The listing builds one solid part. Answer for the finished solid, in the listing's coordinates (mm). Face numbers are marked on the shaded views. A direction names the side the tool comes from. Give positions to 0.01 mm unless a question says otherwise; leave off trailing zeros. Write each loop counter-clockwise with the first axis right and the second up, starting at its lowest first coordinate (ties: lowest second). Pieces come first, ordered by that corner, then holes. Notation, with made-up numbers: (-32.75, 13) - (-2.75, 13) arc R23 ccw to (-2.75, 32) - close; hole circle Ø10 at (69, 54). An arc over 180 degrees is marked (long way). Answer as CSV lines item,"result". Start each with the question number.
(1) Straight lines are drawn through the part: probe 1 along Z at (x, y) = (0, 0.1); probe 2 along Z at (x, y) = (-2, -2.25); probe 3 along Y at (x, z) = (0, 13.25). For each, find the intervals that lie inside material, in ascending order.
(2) Each of these flat-tipped pins is pushed along its axis until it touches: pin 1 Ø3 at (x, z) = (-1, 15) entering from -Y; pin 2 Ø0.7 at (y, z) = (-2, 4) entering from -X; pin 3 Ø0.7 at (y, z) = (-1, 15) entering from +X; pin 4 Ø3 at (x, z) = (0, 15.29) entering from -Y. Where does it stop, or does it pass through?
(3) Find section D-D (x = 2.5). Write down the section's boundary in (y, z), then the cut area to 3 significant figures.
(4) Find section B-B (z = 4). Write down the section's boundary in (x, y), then the cut area to 3 significant figures.
(5) For a pull along X with two mould halves and no side action, classify the marked faces 1, 2 and 3 as pulls with the +X half, pulls with the -X half, needs draft (parallel to the pull), parting line crosses it, or undercut.
(6) Find section A-A (y = -1.4). Write down the section's boundary in (x, z).
(7) Find section C-C (z = 9). Write down the section's boundary in (x, y), then the cut area to 3 significant figures.
(8) For the marked faces 4 and 5, determine the directions among +Z, -Z, +X, -X, +Y, -Y from which every point of the face is accessible in a straight line to the end or side of a thin tool.
from build123d import *

# Parameters (mm, degrees)
PAD_DEPTH       = 20
SKETCH001_W     = 5.88
SKETCH001_H     = 1.68
POCKET_DEPTH    = 20
POCKET001_DEPTH = 2.4
SKETCH003_R     = 1.6
POCKET002_DEPTH = 1.6


with BuildPart() as part:
    # Sketch → Pad (new body)
    with BuildSketch(Plane.XY):
        Polygon((2.94, -2.84), (-2.94, -2.84), (-5.44, -0.52), (-5.44, 1.16), (-2.94, 1.16), (-2.94, 2.84), (2.94, 2.84), (2.94, 1.16), (5.44, 1.16), (5.44, -0.52), align=None)
    extrude(amount=PAD_DEPTH)

    # Sketch001 (on Face11 of Pad) → Pocket (cut)
    with BuildSketch(Plane(origin=(0, 0, 0), x_dir=(1, 0, 0), z_dir=(0, 0, -1))):
        with Locations((0, -2)):
            Rectangle(SKETCH001_W, SKETCH001_H)
    extrude(amount=-POCKET_DEPTH, mode=Mode.SUBTRACT)

    # Sketch002 (on Face1 of Pocket) → Pocket001 (cut)
    with BuildSketch(Plane.XZ.offset(2.84)):
        Polygon((0, 18.6), (-2.87, 16.943005), (-2.87, 13.629014), (0, 11.972019), (2.87, 13.629014), (2.87, 16.943005), align=None)
        Polygon((2.87, 6.370986), (0, 8.027981), (-2.87, 6.370986), (-2.87, 3.056995), (0, 1.4), (2.87, 3.056995), align=None)
    extrude(amount=-POCKET001_DEPTH, mode=Mode.SUBTRACT)

    # Sketch003 (on Face24 of Pocket001) → Pocket002 (cut)
    with BuildSketch(Plane.XZ.offset(0.44)):
        with Locations((0, 15.286009)):
            Circle(SKETCH003_R)
        with Locations((0, 4.713991)):
            Circle(SKETCH003_R)
    extrude(amount=-POCKET002_DEPTH, mode=Mode.SUBTRACT)


solid = part.part
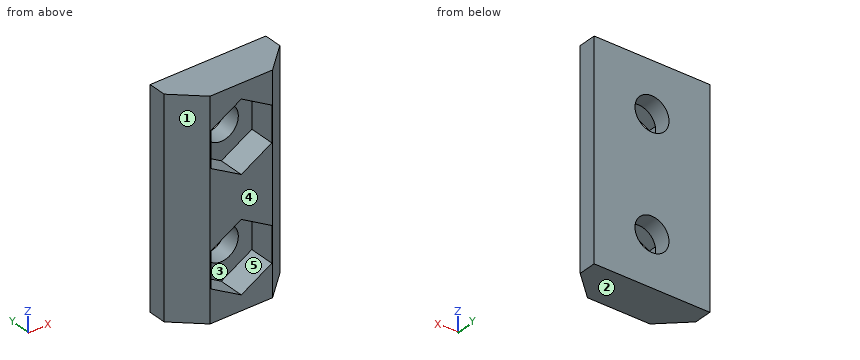
Result set:
1,probe 1,"0 to 3.11, 6.31 to 13.69, 16.89 to 20"
1,probe 2,"0 to 2.55, 6.87 to 13.13, 17.45 to 20"
1,probe 3,"-0.44 to 1.16"
2,pin 1,"y = -0.44"
2,pin 2,"x = -4.22"
2,pin 3,"x = 5.3"
2,pin 4,"through"
3,outline,"(-2.84, 0) - (1.16, 0) - (1.16, 20) - (-2.84, 20) - (-2.84, 17.16) - (-0.44, 17.16) - (-0.44, 13.42) - (-2.84, 13.42) - (-2.84, 6.58) - (-0.44, 6.58) - (-0.44, 2.84) - (-2.84, 2.84) - close"
3,area,"62.0 mm^2"
4,outline,"(-5.44, -0.52) - (-2.94, -2.84) - (-2.87, -2.84) - (-2.87, -0.44) - (-1.43, -0.44) - (-1.43, 1.16) - (-5.44, 1.16) - close; (1.43, -0.44) - (2.87, -0.44) - (2.87, -2.84) - (2.94, -2.84) - (5.44, -0.52) - (5.44, 1.16) - (1.43, 1.16) - close"
4,area,"19.4 mm^2"
5,face 1,"pulls with the -X half"
5,face 2,"needs draft"
5,face 3,"undercut"
6,outline,"(-4.49, 0) - (4.49, 0) - (4.49, 20) - (-4.49, 20) - close; hole (-2.87, 3.06) - (0, 1.4) - (2.87, 3.06) - (2.87, 6.37) - (0, 8.03) - (-2.87, 6.37) - close; hole (-2.87, 13.63) - (0, 11.97) - (2.87, 13.63) - (2.87, 16.94) - (0, 18.6) - (-2.87, 16.94) - close"
7,outline,"(-5.44, -0.52) - (-2.94, -2.84) - (2.94, -2.84) - (5.44, -0.52) - (5.44, 1.16) - (-5.44, 1.16) - close"
7,area,"37.7 mm^2"
8,face 4,"+Z, -Z, +X, -X, -Y"
8,face 5,"-Y"
